Autodesk Inventor part; units mm, degrees
ref_plane "YZ Plane" through (0, 0, 0) normal (1, 0, 0) x (0, 1, 0)
ref_plane "XZ Plane" through (0, 0, 0) normal (0, 1, 0) x (-1, 0, 0)
ref_plane "XY Plane" through (0, 0, 0) normal (0, 0, 1) x (1, 0, 0)
sketch "Sketch1" plane through (0, 0, 0) normal (0, 0, 1) x (1, 0, 0)
  line L0 (-11.2628, -8.9945) -> (-11.2628, -13.0945)
  line L1 (-11.2628, 11.9772) -> (-11.2628, 7.8772)
  line L2 (12.7, 5.5055) -> (12.7, -0.323)
  line L3 (12.7, -6.6945) -> (-7.3, -6.6945)
  line L4 (12.7, 5.5055) -> (-7.3, 5.5055)
  line L5 (-10.4, -1.4801) -> (-10.4, -2.591)
  line L6 (-10.4, 0.291) -> (-10.4, 1.4019)
  line L7 (12.7, -6.6945) -> (-10.4, -6.6945)
  line L8 (-10.4, -6.6945) -> (-10.4, 5.5055)
  line L9 (-10.4, 5.5055) -> (12.7, 5.5055)
  line L10 (12.7, 5.5055) -> (12.7, -6.6945)
  line L11 (12.7, 5.5055) -> (-11.2628, 5.5055)
  line L12 (-11.2628, 5.5055) -> (-11.2628, -6.6945)
  line L13 (-11.2628, -6.6945) -> (12.7, -6.6945)
  line L14 (12.7, -6.6945) -> (12.7, 5.5055)
  line L15 (-11.2628, -0.5945) -> (-12.5719, -0.5945)
  line L16 (-11.2628, -0.5945) -> (13.7372, -0.5945)
  line L17 (13.7372, -0.5945) -> (13.7372, -13.0945)
  line L18 (13.7372, -13.0945) -> (-11.2628, -13.0945)
  line L19 (-11.2628, -13.0945) -> (-11.2628, -0.5945)
  line L20 (13.7372, -0.5945) -> (13.7372, 11.9055)
  line L21 (13.7372, 11.9055) -> (-11.2628, 11.9055)
  line L22 (-11.2628, 11.9055) -> (-11.2628, -0.5945)
  line L23 (11.6, -5.6608) -> (10, -5.6608)
  line L24 (11.6, 5.0392) -> (10, 5.0392)
  line L25 (11.6, 5.0392) -> (11.6, -5.6608)
  line L26 (11.6, 5.0392) -> (10, 5.0392)
  line L27 (10, -5.6608) -> (10, 5.0392)
  line L28 (11.6, -5.6608) -> (10, -5.6608)
  line L29 (11.6, -0.5945) -> (11.6, -5.9445)
  line L30 (11.6, -5.9445) -> (10, -5.9445)
  line L31 (10, -5.9445) -> (10, -0.5945)
  line L32 (11.6, -0.5945) -> (11.6, 4.7555)
  line L33 (11.6, 4.7555) -> (10, 4.7555)
  line L34 (10, 4.7555) -> (10, -0.5945)
  point P0 (0, 0)
  point P1 (-11.2628, -6.6945)
  dimension "d2" = 23.9628
  dimension "d3" = 25
  dimension "d4" = 12.5
  dimension "d5" = 5.35
extrude "Extrusion1" add sketch "Sketch1" along normal blind 1.6 contours L19 L13 L7 L3 L10 L16 L17 L18 L0 | L12 L16 L8 L5 L13 | L12 L11 L8 L6 L16 | L8 L5 L16 L27 L31 L30 L29 L25 L10 L3 L7 | L16 L10 L2 L4 L9 L11 L22 L1 L21 L20 | L8 L6 L9 L4 L2 L10 L16 L25 L24 L27 | L27 L24 L25 L33
properties part number "pcb"
Could you check a few things on this model? Use its own coordinates, in mm. A direction names the side the tool comes from. Give positions to 0.01 mm unless a question says otherwise; leave off trailing zeros. Loops run counter-clockwise (first coordinate to the right, second up) from the corner with the lowest first, then second, coordinate; pieces in that order, holes last. Notation, with made-up numbers: M -26.75,31.25 L -18.75,31.25 A26 cw -18.75,46.25 Z; hole C -36.75,-21 d3. An arc over 180 degrees is marked long. Answer as a JSON object with one key per item and string values.
Q1. For faces 4 (the flat face through (1, 11.906, 1)), 5 (the flat face through (10, -1, 1)), which set-ups out of +Z, -Z, +X, -X, +Y, -Y let a thin tool reach every point of the face, with its end or its side?
Values found:
{"face 4": "+Z, -Z, +X, -X, +Y", "face 5": "+Z, -Z"}
Q2. Suppose I cut it at B-B, the plane z = 0.25. List the corners of the cut face in (x, y) for me, plus the area to 3 significant figures.
Values found:
{"outline": "M -11.26,-13.09 L 13.74,-13.09 L 13.74,11.91 L -11.26,11.91 Z; hole M 10,-5.94 L 11.6,-5.94 L 11.6,4.76 L 10,4.76 Z", "area": "608 mm²"}
Q3. Suppose I cut it at A-A, the plane y = 2.75. List the corners of the cut face in (x, z) for me.
Values found:
{"outline": "M -11.26,0 L 10,0 L 10,1.6 L -11.26,1.6 Z; M 11.6,0 L 13.74,0 L 13.74,1.6 L 11.6,1.6 Z"}
Q4. If I drill on probe 1 along X at (y, z) = (-5.25, 1.4), over which ranges is the centre line in solid material (lowest first)? Write a range as [from, to].
Values found:
{"probe 1": "x = [-11.26, 10], [11.6, 13.74]"}
Q5. If we mould it in two halves opening along X, with no side actions, what happens to faces 1 (the flat face through (1, -13.094, 1)), 2 (the flat face through (11, -5.944, 1)), 3 (the flat face through (-11.263, -1, 1))? For each: pulls with the +X half, pulls with the -X half, needs draft (parallel to the pull), parting line crosses it, or undercut.
Values found:
{"face 1": "needs draft", "face 2": "undercut", "face 3": "pulls with the -X half"}
